Read the model definition and answer for the solid it produces. Units are mm, in the model's axes. Face numbers are marked on the shaded views. A direction names the side the tool comes from. Coordinates: 2 decimals unless noted, no trailing zeros. Loops run counter-clockwise (first coordinate to the right, second up) from the corner with the lowest first, then second, coordinate; pieces in that order, holes last.
Q1. Section C-C (y = -127) is taken. Give the vertices of the cut face in (x, z).
Q2. Straight lines are drawn through the part: line 1 (X direction, y = -54, z = 20.5); line 2 (Y direction, x = 10, z = -31.5); line 3 (Z direction, x = 56.5, y = -33.5). For each, find the intervals that lie inside material, in ascending order.
Q3. Which of the six approach directions +Z, -Z, +X, -X, +Y, -Y give full straight-line access (tool end or side, diameter ignored) to the marked faces 5 and 6?
Q4. The mould has two halves that part along X. Classify the marked faces 1, 2, 3 and 4: pulls with the +X half, pulls with the -X half, needs draft (parallel to the pull), parting line crosses it, or undercut.
Q5. Flat-ended cylindrical pins translate along their axes: P1, Ø5, axis at x = 0, y = -73.5, coming from the +Z side; P2, Ø6, axis at x = 52, z = -27.5, coming from the -Y side. Find the tip coordinate at first contact, or state that the pin passes through.
Q6. Section B-B (x = 65) is taken. Give the vertices of the cut face in (y, z).
Q7. Section A-A (z = -24.5) is taken. Give the vertices of the cut face in (x, y).
from build123d import *

# Parameters (mm, degrees)
F0_W     = 165.1
F0_H     = 114.3
F1_DEPTH = 165.1
F2_T     = -3.81
F3_R     = 10.16


with BuildPart() as f1:
    # F0 (on Front) → F1 (new body)
    with BuildSketch(Plane.XZ):
        Rectangle(F0_W, F0_H)
    extrude(amount=F1_DEPTH)

    # F2
    f2_openings = [f1.faces().sort_by_distance(p)[0] for p in [
        (0, -165.1, 0),
        (0, -82.55, 57.15),
    ]]
    offset(amount=F2_T, openings=f2_openings)

    # F3
    f3_edges = [f1.edges().sort_by_distance(p)[0] for p in [
        (82.55, 0, 0),
        (-82.55, 0, 0),
    ]]
    fillet(f3_edges, radius=F3_R)


solid = f1.part
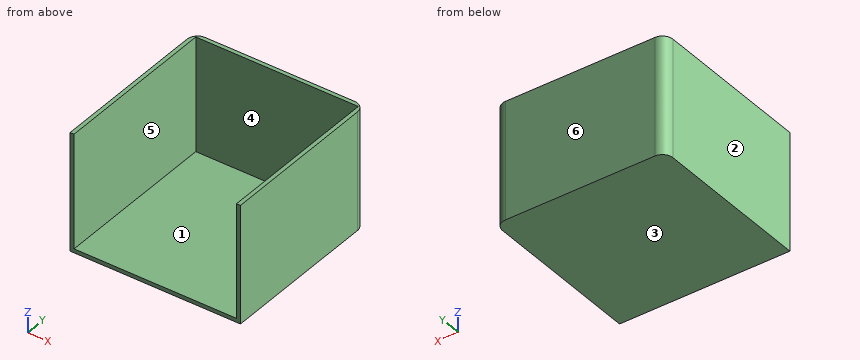
Numbers:
1. outline: (-82.55, -57.15) - (82.55, -57.15) - (82.55, 57.15) - (78.74, 57.15) - (78.74, -53.34) - (-78.74, -53.34) - (-78.74, 57.15) - (-82.55, 57.15) - close
2. line 1: x = -82.55 to -78.74, 78.74 to 82.55
2. line 2: y = -3.81 to 0
2. line 3: z = -57.15 to -53.34
3. face 5: +Z, -Y
3. face 6: +Z, -Z, +X, -X, +Y
4. face 1: undercut
4. face 2: pulls with the -X half
4. face 3: needs draft
4. face 4: undercut
5. P1: stops at z = -53.34
5. P2: stops at y = -3.81
6. outline: (-165.1, -57.15) - (0, -57.15) - (0, 57.15) - (-3.81, 57.15) - (-3.81, -53.34) - (-165.1, -53.34) - close
7. outline: (-82.55, -165.1) - (-78.74, -165.1) - (-78.74, -3.81) - (78.74, -3.81) - (78.74, -165.1) - (82.55, -165.1) - (82.55, -10.16) arc R10.16 ccw to (72.39, 0) - (-72.39, 0) arc R10.16 ccw to (-82.55, -10.16) - close
